from build123d import *

# Parameters (mm, degrees)
ESQUISSE1_W        = 4
ESQUISSE1_H        = 4
BOSS_EXTRU_1_DEPTH = 40
CHANFREIN1_SIZE    = 1


with BuildPart() as part:
    # Esquisse1 → Boss.-Extru.1 (new body)
    with BuildSketch(Plane.XY):
        with Locations((2, 2)):
            Rectangle(ESQUISSE1_W, ESQUISSE1_H)
    extrude(amount=BOSS_EXTRU_1_DEPTH)

    # Chanfrein1
    chanfrein1_edges = [part.edges().sort_by_distance(p)[0] for p in [
        (4, 2, 40),
        (2, 4, 40),
        (0, 2, 40),
        (2, 4, 0),
        (4, 2, 0),
        (2, 0, 0),
        (0, 2, 0),
        (2, 0, 40),
    ]]
    chamfer(chanfrein1_edges, length=CHANFREIN1_SIZE)


solid = part.part
Work out the finished part from the listing and answer in its coordinate system (mm). Round coordinates to 2 decimals unless told otherwise and drop trailing zeros. Write each loop counter-clockwise with the first axis right and the second up, starting at its lowest first coordinate (ties: lowest second). Pieces come first, ordered by that corner, then holes. Notation, with made-up numbers: (32, -20.75) -> (63, -20.75) arc R12 cw to (63, 1.25) -> close; hole circle Ø10 at (-6, 51). An arc over 180 degrees is marked (long way). Answer as CSV lines item,"result". Start each with the question number.
(1) Find the intervals of material crossed by probe 1 along Z at (x, y) = (1.6, 3.7); probe 2 along Z at (x, y) = (0.9, 2), in increasing order.
(2) The part is cut by section A-A, the plane x = 0.6. Give the vertices of the cut face in (y, z).
Output values:
1,probe 1,"z = 0.7 to 39.3"
1,probe 2,"z = 0.1 to 39.9"
2,outline,"(0, 1) -> (0.6, 0.4) -> (3.4, 0.4) -> (4, 1) -> (4, 39) -> (3.4, 39.6) -> (0.6, 39.6) -> (0, 39) -> close"
